Input: part model. Units: mm. Frame: model coordinates. A direction names the side the tool comes from. Give positions to 0.01 mm unless a question says otherwise; leave off trailing zeros. Loops run counter-clockwise (first coordinate to the right, second up) from the corner with the lowest first, then second, coordinate; pieces in that order, holes last. Notation, with made-up numbers: M 26.25,3 L 46.25,3 A12 ccw 46.25,13 Z; hole C -22.5,45 d5. An arc over 180 degrees is marked long. Answer as a JSON object with one key per item and string values. Group by question number.
```python
from build123d import *

# Parameters (mm, degrees)
SKETCH1_W           = 45
SKETCH1_H           = 25.4
BOSS_EXTRUDE1_DEPTH = 8
SKETCH2_W           = 5
SKETCH2_H           = 8
BOSS_EXTRUDE2_DEPTH = 10
SKETCH3_R           = 2
CUT_EXTRUDE1_DEPTH  = 30
LPATTERN1_COUNT     = 2
LPATTERN1_PITCH     = 40
SKETCH4_R           = 1.25
CUT_EXTRUDE2_DEPTH  = 8
LPATTERN2_COUNT     = 2
LPATTERN2_PITCH     = 37


with BuildPart() as part:
    # Sketch1 → Boss-Extrude1 (new body)
    with BuildSketch(Plane(origin=(0, 0, 0), x_dir=(1, 0, 0), z_dir=(0, 1, 0))):
        with Locations((22.5, 12.7)):
            Rectangle(SKETCH1_W, SKETCH1_H)
    extrude(amount=BOSS_EXTRUDE1_DEPTH)

    # Sketch2 → Boss-Extrude2 (add)
    with BuildSketch(Plane.XY):
        with Locations((42.5, 4)):
            Rectangle(SKETCH2_W, SKETCH2_H)
    boss_extrude2 = extrude(amount=BOSS_EXTRUDE2_DEPTH)

    # Sketch3 → Cut-Extrude1 (cut)
    with BuildSketch(Plane.ZY.offset(-40)):
        with Locations((5, 4)):
            Circle(SKETCH3_R)
    cut_extrude1 = extrude(amount=-CUT_EXTRUDE1_DEPTH, mode=Mode.SUBTRACT)

    # LPattern1: Boss-Extrude2, Cut-Extrude1 ×2
    with Locations(*[(-i * LPATTERN1_PITCH, 0, 0) for i in range(1, LPATTERN1_COUNT)]):
        add(boss_extrude2)
        add(cut_extrude1, mode=Mode.SUBTRACT)

    # Sketch4 → Cut-Extrude2 (cut)
    with BuildSketch(Plane.ZY):
        with Locations((-15.4, 4)):
            Circle(SKETCH4_R)
    cut_extrude2 = extrude(amount=-CUT_EXTRUDE2_DEPTH, mode=Mode.SUBTRACT)

    # LPattern2: Cut-Extrude2 ×2
    with Locations(*[(i * LPATTERN2_PITCH, 0, 0) for i in range(1, LPATTERN2_COUNT)]):
        add(cut_extrude2, mode=Mode.SUBTRACT)


solid = part.part
```
1. Section B-B (y = 4). Output: boundary loops of the cut face in (x, z).
2. First-contact query: P1, Ø4.5, axis at y = 4, z = 5, coming from the +X side; P2, Ø3, axis at y = 4, z = 5, coming from the +X side. Flat tips, straight axial feed; report the tip coordinate or a pass-through.
3. Section D-D (y = 6.75). Output: boundary loops of the cut face in (x, z), then the cut area to 3 significant figures.
4. Reachability of faces 4 (the cylindrical face through (3.94, 4.05, -16.65)), 5 (the flat face through (22, 4, 0)), 6 (the flat face through (37, 4, -15)) from +Z, -Z, +X, -X, +Y, -Y: full face, straight path, thin tool, end or side. Return the list, or none.
5. Section C-C (z = -15.4). Output: boundary loops of the cut face in (x, y).
6. Mould query, pull axis X, two halves, no side actions, for faces 1 (the cylindrical face through (42.5, 2.8, 3.4)), 2 (the flat face through (0, 4, -8)), 3 (the flat face through (40, 6, 4)). Classes: pulls with the +X half, pulls with the -X half, needs draft (parallel to the pull), parting line crosses it, or undercut.
7. Material intervals for L1, parallel to Y at x = 41, z = 5; L2, parallel to X at y = 2, z = 8; L3, parallel to Y at x = 5.5, z = -15.4, sorted ascending.
8. Section A-A (z = 5). Output: boundary loops of the cut face in (x, y).
Geometry results:
{
 "1": {"outline": "M 0,-25.4 L 45,-25.4 L 45,-16.65 L 37,-16.65 L 37,-14.15 L 45,-14.15 L 45,3 L 40,3 L 40,0 L 5,0 L 5,3 L 0,3 L 0,-14.15 L 8,-14.15 L 8,-16.65 L 0,-16.65 Z; M 0,7 L 5,7 L 5,10 L 0,10 Z; M 40,7 L 45,7 L 45,10 L 40,10 Z"},
 "2": {"P1": "x = 45", "P2": "through"},
 "3": {"outline": "M 0,-25.4 L 45,-25.4 L 45,10 L 40,10 L 40,0 L 5,0 L 5,10 L 0,10 Z", "area": "1,240 mm2"},
 "4": {"face 4": "-X", "face 5": "+Z, +Y, -Y", "face 6": "+X"},
 "5": {"outline": "M 0,0 L 45,0 L 45,2.75 L 37,2.75 L 37,5.25 L 45,5.25 L 45,8 L 0,8 L 0,5.25 L 8,5.25 L 8,2.75 L 0,2.75 Z"},
 "6": {"face 1": "needs draft", "face 2": "pulls with the -X half", "face 3": "undercut"},
 "7": {"L1": "0 to 2, 6 to 8", "L2": "0 to 5, 40 to 45", "L3": "0 to 2.75, 5.25 to 8"},
 "8": {"outline": "M 0,0 L 5,0 L 5,2 L 0,2 Z; M 0,6 L 5,6 L 5,8 L 0,8 Z; M 40,0 L 45,0 L 45,2 L 40,2 Z; M 40,6 L 45,6 L 45,8 L 40,8 Z"}
}
